Verification items for the finished model (mm, model axes). A direction names the side the tool comes from. Coordinates: 2 decimals unless noted, no trailing zeros. Write each loop counter-clockwise with the first axis right and the second up, starting at its lowest first coordinate (ties: lowest second). Pieces come first, ordered by that corner, then holes. Notation, with made-up numbers: (-7, 73) -> (52, 73) arc R25 cw to (52, 100) -> close; hole circle Ø11 at (65, 70). An arc over 180 degrees is marked (long way). Answer in a Markdown table with one row per item.
```python
from build123d import *

# Parameters (mm, degrees)
BOSS_EXTRUDE1_DEPTH = 3.5
SKETCH2_W           = 9
SKETCH2_H           = 3.5
CUT_EXTRUDE1_DEPTH  = 28.901612857


with BuildPart() as part:
    # Sketch1 → Boss-Extrude1 (new body)
    with BuildSketch(Plane.XY):
        with BuildLine():
            Line((3.5, 26), (3.5, 22.5))
            Line((3.5, 22.5), (1.55, 22.5))
            Line((1.55, 22.5), (1.55, 19.5))
            Line((1.55, 19.5), (2.75, 19.5))
            Line((2.75, 19.5), (2.75, 17))
            Line((2.75, 17), (1.55, 17))
            Line((1.55, 17), (1.55, 13.5))
            Line((1.55, 13.5), (-1.55, 13.5))
            Line((-1.55, 13.5), (-1.55, 17))
            Line((-1.55, 17), (-2.75, 17))
            Line((-2.75, 17), (-2.75, 19.5))
            Line((-2.75, 19.5), (-1.55, 19.5))
            Line((-1.55, 19.5), (-1.55, 22.5))
            Line((-1.55, 22.5), (-3.5, 22.5))
            Line((-3.5, 22.5), (-3.5, 26))
            Line((-3.5, 26), (-9.5, 26))
            Line((-9.5, 26), (-9.5, -26))
            Line((-9.5, -26), (-3.5, -26))
            Line((-3.5, -26), (-3.5, -22.5))
            Line((-3.5, -22.5), (-1.55, -22.5))
            Line((-1.55, -22.5), (-1.55, -19.5))
            Line((-1.55, -19.5), (-2.75, -19.5))
            Line((-2.75, -19.5), (-2.75, -17))
            Line((-2.75, -17), (-1.55, -17))
            Line((-1.55, -17), (-1.55, -13.5))
            Line((-1.55, -13.5), (1.55, -13.5))
            Line((1.55, -13.5), (1.55, -17))
            Line((1.55, -17), (2.75, -17))
            Line((2.75, -17), (2.75, -19.5))
            Line((2.75, -19.5), (1.55, -19.5))
            Line((1.55, -19.5), (1.55, -22.5))
            Line((1.55, -22.5), (3.5, -22.5))
            Line((3.5, -22.5), (3.5, -26))
            Line((3.5, -26), (9.5, -26))
            Line((9.5, -26), (9.5, -21))
            ThreePointArc((9.5, -21), (5, -15.175053648), (9.5, -9.350107297))
            Line((9.5, -9.350107297), (9.5, 9.350107297))
            ThreePointArc((9.5, 9.350107297), (5, 15.175053648), (9.5, 21))
            Line((9.5, 21), (9.5, 26))
            Line((9.5, 26), (3.5, 26))
        make_face()
    extrude(amount=BOSS_EXTRUDE1_DEPTH)

    # Sketch2 → Cut-Extrude1 (cut, through all)
    with BuildSketch(Plane.XY.offset(3.5)):
        with Locations((1, 0.25)):
            Rectangle(SKETCH2_W, SKETCH2_H)
    extrude(amount=-CUT_EXTRUDE1_DEPTH, mode=Mode.SUBTRACT)


solid = part.part
```
1. Go/stop test with flat-tipped pins: pin 1 (1.5 mm diameter, centred on x = -0.5, z = 1, fed in from +Y); pin 2 (1 mm diameter, centred on x = -2, z = 1.5, fed in from -Y); pin 3 (1.5 mm diameter, centred on x = 2.5, z = 2, fed in from +Y). Record where each tip stops, or that it passes through.
Findings below:
| item | result |
|---|---|
| pin 1 | stops at y = 13.5 |
| pin 2 | stops at y = -22.5 |
| pin 3 | stops at y = 22.5 |
2. Access from +Z, -Z, +X, -X, +Y, -Y to the whole of each face (thin tool, end or side, straight path). Record for faces 1 (the face through (-1.55, 15, 2)), 2 (the face through (0, -13.5, 2)), 3 (the face through (-2, -17, 2)).
Findings below:
| item | result |
|---|---|
| face 1 | +Z, -Z, +Y |
| face 2 | +Z, -Z, -Y |
| face 3 | +Z, -Z |
3. Sectioned sample at A-A, the plane x = 1. Record the cut outline in (y, z).
Findings below:
| item | result |
|---|---|
| outline | (-13.5, 0) -> (-1.5, 0) -> (-1.5, 3.5) -> (-13.5, 3.5) -> close; (2, 0) -> (13.5, 0) -> (13.5, 3.5) -> (2, 3.5) -> close |
4. Release check for a two-part mould opening along Y. For faces 4 (the face through (-2.75, 18, 2)), 5 (the face through (-1.55, 21, 2)), 6 (the face through (3, -22.5, 2)) record: released by +Y, released by -Y, zero draft, split by the parting line, or undercut.
Findings below:
| item | result |
|---|---|
| face 4 | undercut |
| face 5 | zero draft |
| face 6 | released by -Y |
5. Sectioned sample at B-B, the plane y = 14.5. Record the cut outline in (x, z), and give its area (3 significant figures).
Findings below:
| item | result |
|---|---|
| outline | (-9.5, 0) -> (-1.55, 0) -> (-1.55, 3.5) -> (-9.5, 3.5) -> close; (1.55, 0) -> (5.04, 0) -> (5.04, 3.5) -> (1.55, 3.5) -> close |
| area | 40.0 mm² |
6. Material ranges on probe 1 along Y at (x, z) = (-2, 0.45); probe 2 along X at (y, z) = (0, 0.8); probe 3 along Y at (x, z) = (8.25, 1.2), recorded low to high. Write a range as from..to.
Findings below:
| item | result |
|---|---|
| probe 1 | y = -22.5..-19.5, -17..-1.5, 2..17, 19.5..22.5 |
| probe 2 | x = -9.5..-3.5, 5.5..9.5 |
| probe 3 | y = -26..-20.52, -9.83..9.83, 20.52..26 |
